Could you check a few things on this model? Use its own coordinates, in mm. A direction names the side the tool comes from. Give positions to 0.01 mm unless a question says otherwise; leave off trailing zeros. Write each loop counter-clockwise with the first axis right and the second up, starting at its lowest first coordinate (ties: lowest second). Pieces come first, ordered by that corner, then holes. Notation, with made-up numbers: M -15,58 L 12,58 A30 ccw 12,87 Z; hole C 76.5,-32 d5. An arc over 180 degrees is marked long. Use one line per item in the form item = value.
Solid Edge part; units mm, degrees
sketch "Sketch1" plane through (0, 0, 0) normal (0, -1, 0) x (1, 0, 0)
  line L0 (25, 129.6172) -> (42.2199, 3)
  line L1 (50, 3) -> (42.2199, 3)
  line L2 (50, 0) -> (50, 3)
  line L3 (50, 0) -> (70, 0)
  line L4 (70, 0) -> (70, 20)
  line L5 (70, 20) -> (50, 20)
  line L6 (33, 145) -> (50, 20)
  line L7 (35, 145) -> (33, 145)
  line L8 (35, 185) -> (35, 145)
  line L9 (25, 185) -> (35, 185)
  line L10 (25, 185) -> (25, 129.6172)
  dimension "D1" = 35
  dimension "D2" = 50
  dimension "D3" = 70
  dimension "D4" = 70
  dimension "D5" = 35
  dimension "D6" = 35
revolve "RevolvedProtrusion1" add sketch "Sketch1" angle 360 about axis through (0, 0, 54) along (0, 0, -1)
fillet "Round1" radius 1 1 edges at (-50, 0, 3)
fillet "Round_2" radius 8 1 edges at (-50, 0, 20)
fillet "Round_3" radius 1 1 edges at (-35, 0, 145)
1) If I drill on L1, parallel to X at y = 0, z = 1.3; L2, parallel to Y at x = 0, z = 170, over which ranges is the centre line in solid material (lowest first)?
Checked values:
L1 = -70 to -50, 50 to 70
L2 = -35 to -25, 25 to 35
2) Thinking about a two-plate mould opening in Y: for faces 4 (the flat face through (-24, -8, 185)), 5 (the flat face through (22, -37, 3)), 6 (the cylindrical face through (-55.55, -42.594, 10.14)), which applies, released by +Y, released by -Y, zero draft, split by the parting line, or undercut?
Checked values:
face_4 = zero draft
face_5 = undercut
face_6 = split by the parting line
3) For pin 1 Ø3 at (x, z) = (-22, 109.5) entering from +Y; pin 2 Ø12 at (y, z) = (30, 136.5) entering from +X; pin 3 Ø1.5 at (x, y) = (-39, 51.5) entering from +Z, each with a flat end and sliding along its axis, tell me the tip position at first contact or that it passes through.
Checked values:
pin_1 = 31.82
pin_2 = 24.41
pin_3 = 20
4) For faces 1 (the flat face through (-28, -18, 145)), 2 (the cylindrical face through (47.69, 15.02, 1.01)), 3 (the flat face through (-57.4, -0.3, 20)), which set-ups out of +Z, -Z, +X, -X, +Y, -Y let a thin tool reach every point of the face, with its end or its side?
Checked values:
face_1 = none
face_2 = -Z
face_3 = +Z
5) I want a section at A-A, the plane y = 0. Please give me the cut outline in (x, z).
Checked values:
outline = M -70,0 L -50,0 L -50,2 A1 cw -49,3 L -42.22,3 L -25,129.62 L -25,185 L -35,185 L -35,146 A1 ccw -34,145 L -33,145 L -49.06,26.92 A8 cw -56.99,20 L -70,20 Z; M 25,129.62 L 42.22,3 L 49,3 A1 cw 50,2 L 50,0 L 70,0 L 70,20 L 56.99,20 A8 cw 49.06,26.92 L 33,145 L 34,145 A1 ccw 35,146 L 35,185 L 25,185 Z
6) I want a section at C-C, the plane z = 31. Please give me the cut outline in (x, y).
Checked values:
outline = C 0,0 d97.01; hole C 0,0 d76.82
7) I want a section at D-D, the plane z = 116.5. Please give me the cut outline in (x, y), plus the area to 3 significant figures.
Checked values:
outline = C 0,0 d73.75; hole C 0,0 d53.57
area = 2,020 mm2
